Geometry: final body of the model. Coordinates: model frame, mm. Face numbers are marked on the shaded views. A direction names the side the tool comes from. Round coordinates to 2 decimals unless told otherwise and drop trailing zeros. Order: outer loops, then holes, each group sorted by start corner. A loop starts at its lowest first (then second) coordinate and runs counter-clockwise, first axis right, second up. Notation, with made-up numbers: (24, 76.25) - (45, 76.25) arc R33 cw to (45, 112.25) - close; hole circle Ø10 at (-8.75, -28.75). An arc over 180 degrees is marked (long way). Put each result on its own line as item: value. Start each with the question number.
(1) Pin query (flat end, axial travel): P1, Ø1, axis at x = 198, z = 242, coming from the -Y side; P2, Ø6, axis at y = 108.5, z = 269, coming from the +X side; P3, Ø1.5, axis at x = -267, z = 62.5, coming from the +Y side. Return the tip coordinate at first contact, or that it passes through.
(2) Access query for the marked faces 1, 2 and 3. Directions: +Z, -Z, +X, -X, +Y, -Y. A direction counts if a zero-diameter tool reaches every point of the face in a straight line with its end or side. Return the directions, or none.
(3) Material intervals for L1, parallel to Y at x = -150, z = 207; L2, parallel to X at y = 76, z = 209.5; L3, parallel to X at y = 155, z = 211.5, sorted ascending. Write a range as [from, to].
(4) Pull-direction query (Y, two-part tool) for the marked faces 4, 5, 6 and 7; classes: released by +Y, released by -Y, zero draft, split by the parting line, or undercut.
(5) Section A-A (x = -144). Output: boundary loops of the cut face in (y, z), and give its area (3 significant figures).
(6) Section C-C (x = 213). Output: boundary loops of the cut face in (y, z).
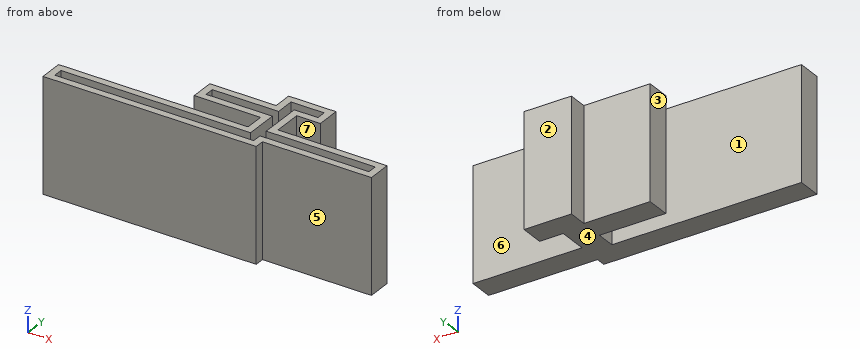
from build123d import *

# Parameters (mm, degrees)
BOSS_EXTRUDE1_DEPTH = 304.8
SHELL1_T            = -19.05


with BuildPart() as part:
    # Sketch1 → Boss-Extrude1 (new body)
    with BuildSketch(Plane.XY):
        Polygon((-241.3, 177.8), (-63.5, 177.8), (-63.5, 228.6), (63.5, 228.6), (63.5, 165.1), (0, 165.1), (0, 88.9), (292.1, 88.9), (292.1, 25.4), (0, 25.4), (0, 0), (-571.5, 0), (-571.5, 63.5), (-63.5, 63.5), (-63.5, 114.3), (-241.3, 114.3), align=None)
    extrude(amount=BOSS_EXTRUDE1_DEPTH)

    # Shell1
    shell1_openings = [part.faces().sort_by_distance(p)[0] for p in [
        (-152.4, 168.866563259, 304.8),
    ]]
    offset(amount=SHELL1_T, openings=shell1_openings, kind=Kind.INTERSECTION)


solid = part.part
Checks:
1. P1: stops at y = 25.4
1. P2: stops at x = 0
1. P3: stops at y = 63.5
2. face 1: +Z, -Z, -X
2. face 2: +Z, -Z, +X, -X, +Y
2. face 3: +Z, -Z, -X, +Y
3. L1: y = [0, 19.05], [44.45, 63.5], [114.3, 133.35], [158.75, 177.8]
3. L2: x = [-63.5, -44.45], [-19.05, 292.1]
3. L3: x = [-241.3, -222.25], [-19.05, 0]
4. face 4: zero draft
4. face 5: released by -Y
4. face 6: undercut
4. face 7: undercut
5. outline: (0, 0) - (63.5, 0) - (63.5, 304.8) - (44.45, 304.8) - (44.45, 19.05) - (19.05, 19.05) - (19.05, 304.8) - (0, 304.8) - close; (114.3, 0) - (177.8, 0) - (177.8, 304.8) - (158.75, 304.8) - (158.75, 19.05) - (133.35, 19.05) - (133.35, 304.8) - (114.3, 304.8) - close
5. area: 24,200 mm²
6. outline: (25.4, 0) - (88.9, 0) - (88.9, 304.8) - (69.85, 304.8) - (69.85, 19.05) - (44.45, 19.05) - (44.45, 304.8) - (25.4, 304.8) - close
